```python
from build123d import *

# Parameters (mm, degrees)
SKIZZE1_R                       = 21.75
SKIZZE1_R_2                     = 2
SKIZZE1_R_3                     = 6
AUFSATZ_LINEAR_AUSTRAGEN1_DEPTH = 1


with BuildPart() as part:
    # Skizze1 → Aufsatz-Linear austragen1 (new body)
    with BuildSketch(Plane.XY):
        Circle(SKIZZE1_R)
        with Locations((11.75, 0)):
            Circle(SKIZZE1_R_2, mode=Mode.SUBTRACT)
        with Locations((5.875, -10.175798494)):
            Circle(SKIZZE1_R_2, mode=Mode.SUBTRACT)
        with Locations((-5.875, -10.175798494)):
            Circle(SKIZZE1_R_2, mode=Mode.SUBTRACT)
        with Locations((-11.75, 0)):
            Circle(SKIZZE1_R_2, mode=Mode.SUBTRACT)
        with Locations((-5.875, 10.175798494)):
            Circle(SKIZZE1_R_2, mode=Mode.SUBTRACT)
        with Locations((5.875, 10.175798494)):
            Circle(SKIZZE1_R_2, mode=Mode.SUBTRACT)
        Circle(SKIZZE1_R_3, mode=Mode.SUBTRACT)
    extrude(amount=AUFSATZ_LINEAR_AUSTRAGEN1_DEPTH)


solid = part.part
```
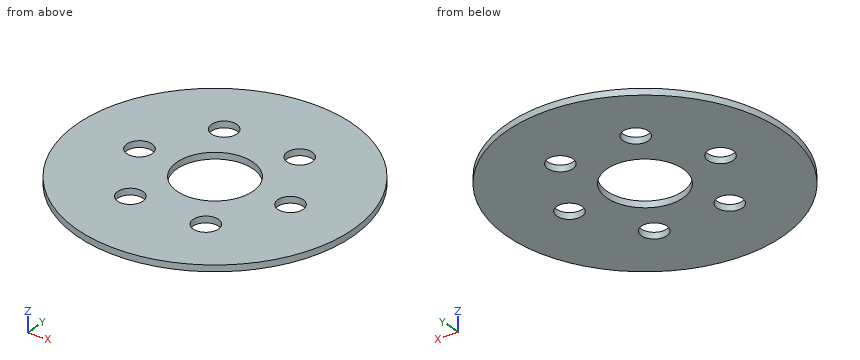
CAD build for the part. Positions are in the model's coordinates, mm. Round coordinates to 2 decimals unless told otherwise and drop trailing zeros. Order: outer loops, then holes, each group sorted by start corner. A loop starts at its lowest first (then second) coordinate and runs counter-clockwise, first axis right, second up.
Item 1: Saw through at B-B on y = 0. Write the cut outline in (x, z), then the cut area to 3 significant figures.
Item 2: Probe line 1 along X through (y, z) = (-12, 0.35); line 2 along X through (y, z) = (-9, 0.75); line 3 along Y through (x, z) = (5, 0.7). List the from-to ranges inside material, lowest first.
Item 3: Pin check, flat tips, straight feed: pin 1 (4.5 mm diameter, centred on x = -5.88, y = -10.18, fed in from -Z); pin 2 (2.5 mm diameter, centred on x = 5.88, y = -10.18, fed in from -Z). Stop position of each tip, or through.
Item 4: Saw through at A-A on x = 0. Write the cut outline in (y, z), then the cut area to 3 significant figures.
Item 5: Saw through at D-D on x = 12. Write the cut outline in (y, z).
Item 6: Saw through at C-C on z = 0.5. Write the cut outline in (x, y) (3 decimals).
Reported:
1. outline: (-21.75, 0) - (-13.75, 0) - (-13.75, 1) - (-21.75, 1) - close; (-9.75, 0) - (-6, 0) - (-6, 1) - (-9.75, 1) - close; (6, 0) - (9.75, 0) - (9.75, 1) - (6, 1) - close; (13.75, 0) - (21.75, 0) - (21.75, 1) - (13.75, 1) - close
1. area: 23.5 mm2
2. line 1: x = -18.14 to -6.69, -5.06 to 5.06, 6.69 to 18.14
2. line 2: x = -19.8 to -7.49, -4.26 to 4.26, 7.49 to 19.8
2. line 3: y = -21.17 to -11.97, -8.38 to -3.32, 3.32 to 8.38, 11.97 to 21.17
3. pin 1: stops at z = 0
3. pin 2: passes through
4. outline: (-21.75, 0) - (-6, 0) - (-6, 1) - (-21.75, 1) - close; (6, 0) - (21.75, 0) - (21.75, 1) - (6, 1) - close
4. area: 31.5 mm2
5. outline: (-18.14, 0) - (-1.98, 0) - (-1.98, 1) - (-18.14, 1) - close; (1.98, 0) - (18.14, 0) - (18.14, 1) - (1.98, 1) - close
6. outline: circle Ø43.5 at (0, 0); hole circle Ø4 at (-11.75, 0); hole circle Ø4 at (-5.875, -10.176); hole circle Ø4 at (-5.875, 10.176); hole circle Ø12 at (0, 0); hole circle Ø4 at (5.875, -10.176); hole circle Ø4 at (5.875, 10.176); hole circle Ø4 at (11.75, 0)
